Input: part model. Units: mm. Frame: model coordinates. A direction names the side the tool comes from. Coordinates: 2 decimals unless noted, no trailing zeros. Write each loop counter-clockwise with the first axis right and the second up, starting at its lowest first coordinate (ties: lowest second). Pieces come first, ordered by that corner, then holes. Notation, with made-up numbers: (-26, 12) - (-7, 12) arc R30 cw to (-7, 37) - close; hole circle Ø6 at (29, -34). An arc over 180 degrees is marked (long way). Use a Markdown table: item, result. Add a question column.
Q1. Section query B-B (y = 0). Return the cut outline in (x, z) (3 decimals).
Q2. Material intervals for probe 1 along Y at (x, z) = (3.25, 0) (3 decimals); probe 2 along X at (y, z) = (11.25, 0); probe 3 along Z at (x, y) = (11, -3), sorted ascending. Write a range as from..to.
Q3. Mould query, pull axis Z, two halves, no side actions, for faces 3 (the face through (12.7, -7, -7)), 4 (the face through (0.18, -9.3, 2.06)), 5 (the face through (0.178, -15.497, 3.441)). Classes: released by +Z, released by -Z, zero draft, split by the parting line, or undercut.
Q4. Section query D-D (x = -4.25). Return the cut outline in (y, z) (3 decimals), then the cut area to 3 significant figures.
Q5. Set-up query: faces 1 (the face through (0.71, 12.562, -1.713)), 2 (the face through (-12.7, -7, -7)). Return all of +Z, -Z, +X, -X, +Y, -Y with unobstructed straight access to the full face (end or side cutting, diameter ignored); none if empty.
Q6. Section query A-A (z = 0). Return the cut outline in (x, y) (3 decimals).
Q7. Pin query (flat end, axial travel): P1, Ø12, axis at x = -3.5, y = -9, coming from the +Z side; P2, Ø2, axis at x = 4.5, y = -7.5, coming from the -Z side; P3, Ø1, axis at x = 6.5, y = 12, coming from the -Z side. Return the tip coordinate at first contact, or that it passes through.
Q8. Section query C-C (z = -8). Return the cut outline in (x, y), then the cut area to 3 significant figures.
from build123d import *

# Parameters (mm, degrees)
SKETCH1_R           = 15.875
BOSS_EXTRUDE1_DEPTH = 12.7
SKETCH2_R           = 9.525
F_3_4_REAM_DEPTH    = 34.89972345
SKETCH3_R           = 1.8542
F_10_32_TAP_DEPTH   = 26.793821935


with BuildPart() as part:
    # Sketch1 → Boss-Extrude1 (new, symmetric)
    with BuildSketch(Plane(origin=(0, 0, 0), x_dir=(0, 0, -1), z_dir=(1, 0, 0))):
        Circle(SKETCH1_R)
    extrude(amount=BOSS_EXTRUDE1_DEPTH, both=True)

    # Sketch2 → 3/4 Ream (cut, through all)
    with BuildSketch(Plane(origin=(12.7, 0, 0), x_dir=(0, 0, -1), z_dir=(1, 0, 0))):
        Circle(SKETCH2_R)
    extrude(amount=-F_3_4_REAM_DEPTH, mode=Mode.SUBTRACT)

    # Sketch3 → #10-32 Tap (cut, through all)
    with BuildSketch(Plane(origin=(0, 0, 0), x_dir=(1, 0, 0), z_dir=(0, 1, 0))):
        with Locations(Location((0, 0, 0), (0, 0, 90))):
            Circle(SKETCH3_R)
    extrude(amount=F_10_32_TAP_DEPTH, mode=Mode.SUBTRACT)


solid = part.part
Values follow:
| question | item | result |
|---|---|---|
| 1 | outline | (-12.7, -15.875) - (12.7, -15.875) - (12.7, -9.525) - (-12.7, -9.525) - close; (-12.7, 9.525) - (12.7, 9.525) - (12.7, 15.875) - (-12.7, 15.875) - close |
| 2 | probe 1 | -15.875..-9.525, 9.525..15.875 |
| 2 | probe 2 | -12.7..-1.85, 1.85..12.7 |
| 2 | probe 3 | -15.59..-9.04, 9.04..15.59 |
| 3 | face 3 | zero draft |
| 3 | face 4 | undercut |
| 3 | face 5 | split by the parting line |
| 4 | outline | circle Ø31.75 at (0, 0); hole circle Ø19.05 at (0, 0) |
| 4 | area | 507 mm2 |
| 5 | face 1 | +Y |
| 5 | face 2 | +Z, -Z, -X, +Y, -Y |
| 6 | outline | (-12.7, -15.875) - (12.7, -15.875) - (12.7, -9.525) - (-12.7, -9.525) - close; (-12.7, 9.525) - (-1.854, 9.525) - (-1.854, 15.875) - (-12.7, 15.875) - close; (1.854, 9.525) - (12.7, 9.525) - (12.7, 15.875) - (1.854, 15.875) - close |
| 7 | P1 | z = 15.59 |
| 7 | P2 | z = -14.48 |
| 7 | P3 | z = -10.94 |
| 8 | outline | (-12.7, -13.71) - (12.7, -13.71) - (12.7, -5.17) - (-12.7, -5.17) - close; (-12.7, 5.17) - (12.7, 5.17) - (12.7, 13.71) - (-12.7, 13.71) - close |
| 8 | area | 434 mm2 |
